Read the model definition and answer for the solid it produces. Units are mm, in the model's axes. A direction names the side the tool comes from. Round coordinates to 2 decimals unless told otherwise and drop trailing zeros. Order: outer loops, then holes, each group sorted by start corner. A loop starts at its lowest first (then second) coordinate and runs counter-clockwise, first axis right, second up. Notation, with made-up numbers: (-20.75, 11) -> (1.25, 11) arc R14 cw to (1.25, 36) -> close; hole circle Ø6 at (-9, -31). An arc over 180 degrees is marked (long way). One line per item, written item: value. Start each with the question number.
1. Flat-ended cylindrical pins translate along their axes: pin 1 Ø0.5 at (y, z) = (-2.5, -5) entering from -X; pin 2 Ø1.5 at (y, z) = (-0.5, -4.5) entering from -X (3 decimals); pin 3 Ø1.5 at (x, y) = (-3, -3) entering from +Z; pin 4 Ø0.5 at (y, z) = (-2, -2.5) entering from +X. Find the tip coordinate at first contact, or state that the pin passes through.
2. The mould has two halves that part along X. Classify faces 1 (the face through (0, 3, -6.45)), 2 (the face through (-3.3, 5.86, 2.9)), 3 (the face through (-4.815, 3, 0)): released by +X, released by -X, zero draft, split by the parting line, or undercut.
3. Section B-B (y = -3.75) is taken. State how many separate pieces and enclosed holes the cut face has, then the cut area to 3 significant figures.
4. For faces 4 (the face through (4.815, 3, 0)), 5 (the face through (-3.8, 5.86, -5.5)), 6 (the face through (0, 0.5, 0)), determine the directions among +Z, -Z, +X, -X, +Y, -Y from which every point of the face is accessible in a straight line to the end or side of a thin tool.
5. Consider line 1 (X direction, y = -1.5, z = 5); line 2 (Y direction, x = -0.5, z = 5.75); line 3 (Y direction, x = 3.5, z = 1.25). Determine where each line is inside the solid, lowest interval first.
6. Section A-A (x = -0.75) is taken. Give the vertices of the cut face in (y, z), then the cut area to 3 significant figures.
from build123d import *

# Parameters (mm, degrees)
SKETCH1_W           = 9.63
SKETCH1_H           = 12.9
BOSS_EXTRUDE1_DEPTH = 6.36
SKETCH2_W           = 6
SKETCH2_H           = 12.9
CUT_EXTRUDE1_DEPTH  = 0.5
FILLET1_R           = 0.5
SKETCH3_W           = 0.64
SKETCH3_H           = 0.64
BOSS_EXTRUDE2_DEPTH = 5
SKETCH4_R           = 0.4
CUT_EXTRUDE2_DEPTH  = 0.5


with BuildPart() as part:
    # Sketch1 → Boss-Extrude1 (new body)
    with BuildSketch(Plane(origin=(0, 0, 0), x_dir=(1, 0, 0), z_dir=(0, 1, 0))):
        Rectangle(SKETCH1_W, SKETCH1_H)
    extrude(amount=BOSS_EXTRUDE1_DEPTH)

    # Sketch2 → Cut-Extrude1 (cut)
    with BuildSketch(Plane.XZ):
        Rectangle(SKETCH2_W, SKETCH2_H)
    extrude(amount=-CUT_EXTRUDE1_DEPTH, mode=Mode.SUBTRACT)

    # Fillet1
    fillet1_edges = [part.edges().sort_by_distance(p)[0] for p in [
        (3, 0, 0),
        (-3, 0, 0),
    ]]
    fillet(fillet1_edges, radius=FILLET1_R - 0.0001)  # a hair under: the kernel refuses the full size

    # Sketch3 → Boss-Extrude2 (add)
    with BuildSketch(Plane.XZ):
        with Locations((-3.81, 2.54)):
            Rectangle(SKETCH3_W, SKETCH3_H)
        with Locations((-3.81, 5.08)):
            Rectangle(SKETCH3_W, SKETCH3_H)
        with Locations((-3.81, 0)):
            Rectangle(SKETCH3_W, SKETCH3_H)
        with Locations((-3.81, -2.54)):
            Rectangle(SKETCH3_W, SKETCH3_H)
        with Locations((-3.81, -5.08)):
            Rectangle(SKETCH3_W, SKETCH3_H)
        with Locations((3.81, 2.54)):
            Rectangle(SKETCH3_W, SKETCH3_H)
        with Locations((3.81, 5.08)):
            Rectangle(SKETCH3_W, SKETCH3_H)
        with Locations((3.81, 0)):
            Rectangle(SKETCH3_W, SKETCH3_H)
        with Locations((3.81, -2.54)):
            Rectangle(SKETCH3_W, SKETCH3_H)
        with Locations((3.81, -5.08)):
            Rectangle(SKETCH3_W, SKETCH3_H)
    extrude(amount=BOSS_EXTRUDE2_DEPTH)

    # Sketch4 → Cut-Extrude2 (cut)
    with BuildSketch(Plane(origin=(0, 6.36, 0), x_dir=(1, 0, 0), z_dir=(0, 1, 0))):
        with Locations(Location((-3.796432961, 5.485774113, 0), (0, 0, 270))):
            Circle(SKETCH4_R)
        Polygon((3.97982075, 4.592848347), (3.28522804, 0.653617335), (2.706000074, 0.248037547), (2.300420287, 0.827265513), (2.995012997, 4.766496525), (3.574240963, 5.172076312), align=None)
        Polygon((2.981343729, -1.069796233), (2.286751018, -5.009027245), (1.703567039, -5.41390948), (1.296354761, -4.832350077), (1.990947472, -0.893119065), (2.574131451, -0.48823683), align=None)
        Polygon((-3.021593907, -4.95), (0.978406093, -4.95), (1.476350329, -5.45), (0.978406093, -5.95), (-3.021593907, -5.95), (-3.519538144, -5.45), align=None)
        Polygon((-2.208030846, 0.350112276), (1.991969154, 0.350112276), (2.477076686, -0.136998017), (1.991969154, -0.62410831), (-2.208030846, -0.62410831), (-2.693138379, -0.136998017), align=None)
        Polygon((-1.254148002, 5.95), (2.745851998, 5.95), (3.31109238, 5.485774113), (2.813148144, 4.95), (-1.186851856, 4.95), (-1.752092238, 5.414225887), align=None)
        Polygon((-2.518656271, -1.069796233), (-3.213248982, -5.009027245), (-3.796432961, -5.41390948), (-4.203645239, -4.832350077), (-3.509052528, -0.893119065), (-2.925868549, -0.48823683), align=None)
        Polygon((-1.925759037, 5.172076312), (-1.52017925, 4.592848347), (-2.21477196, 0.653617335), (-2.793999926, 0.248037547), (-3.199579713, 0.827265513), (-2.504987003, 4.766496525), align=None)
    extrude(amount=-CUT_EXTRUDE2_DEPTH, mode=Mode.SUBTRACT)


solid = part.part
Answer:
1. pin 1: x = -4.13
1. pin 2: x = -4.815
1. pin 3: z = 5.4
1. pin 4: x = 4.13
2. face 1: zero draft
2. face 2: undercut
2. face 3: released by -X
3. separate pieces: 10
3. enclosed holes: 0
3. area: 4.10 mm^2
4. face 4: +Z, -Z, +X, +Y, -Y
4. face 5: +Y
4. face 6: +Z, -Z, -Y
5. line 1: -4.13 to -3.49, 3.49 to 4.13
5. line 2: 0.5 to 5.86
5. line 3: 0 to 6.36
6. outline: (0.5, -6.45) -> (6.36, -6.45) -> (6.36, -5.95) -> (5.86, -5.95) -> (5.86, -4.95) -> (6.36, -4.95) -> (6.36, -0.35) -> (5.86, -0.35) -> (5.86, 0.62) -> (6.36, 0.62) -> (6.36, 4.95) -> (5.86, 4.95) -> (5.86, 5.95) -> (6.36, 5.95) -> (6.36, 6.45) -> (0.5, 6.45) -> close
6. area: 74.1 mm^2
